from build123d import *

# Parameters (mm, degrees)
SKETCH1_W           = 90
SKETCH1_H           = 60
BOSS_EXTRUDE1_DEPTH = 5
SKETCH2_R           = 1.1
SKETCH2_R_2         = 0.62
SKETCH2_R_3         = 0.6858
SKETCH2_R_4         = 0.5
CUT_EXTRUDE1_DEPTH  = 61
SKETCH3_R           = 2
CUT_EXTRUDE2_DEPTH  = 6


with BuildPart() as part:
    # Sketch1 → Boss-Extrude1 (new body)
    with BuildSketch(Plane(origin=(0, 0, 0), x_dir=(1, 0, 0), z_dir=(0, 1, 0))):
        with Locations((-15.754716981, 62.075471698)):
            Rectangle(SKETCH1_W, SKETCH1_H)
    extrude(amount=BOSS_EXTRUDE1_DEPTH)

    # Sketch2 → Cut-Extrude1 (cut, through all)
    with BuildSketch(Plane.XY.offset(-32.075471698)):
        with Locations((-45.754716981, 5.25)):
            Circle(SKETCH2_R)
        with Locations((-25.754716981, 5.25)):
            Circle(SKETCH2_R_2)
        with Locations((-5.754716981, 5.25)):
            Circle(SKETCH2_R_3)
        with Locations((14.245283019, 5.25)):
            Circle(SKETCH2_R_4)
    extrude(amount=-CUT_EXTRUDE1_DEPTH, mode=Mode.SUBTRACT)

    # Sketch3 → Cut-Extrude2 (cut, through all)
    with BuildSketch(Plane(origin=(0, 5, 0), x_dir=(1, 0, 0), z_dir=(0, 1, 0))):
        with Locations((-53.907444579, 80.442311963)):
            Circle(SKETCH3_R)
        with Locations((-43.907444579, 80.442311963)):
            Circle(SKETCH3_R)
    extrude(amount=-CUT_EXTRUDE2_DEPTH, mode=Mode.SUBTRACT)


solid = part.part
Geometry check sheet. Reference: the model listing, model coordinates, mm. Round coordinates to 2 decimals unless told otherwise and drop trailing zeros. Write each loop counter-clockwise with the first axis right and the second up, starting at its lowest first coordinate (ties: lowest second). Pieces come first, ordered by that corner, then holes. Notation, with made-up numbers: (50, 41) -> (65, 41) arc R27 cw to (65, 61) -> close; hole circle Ø7 at (20, -7.5). An arc over 180 degrees is marked (long way). One line per item, written item: value. Start each with the question number.
(1) Draft check along X on faces 1 (the flat face through (29.245, 2, -62)), 2 (the cylindrical face through (-55.382, 2.535, -81.794)), 3 (the flat face through (-16, 2, -32.075)). Enter one of: +X half, -X half, draft (parallel to the pull), parting line (faces both ways), or undercut.
(2) Scan lines: line 1 (X direction, y = 2.7, z = -81); line 2 (X direction, y = 4.25, z = -66.5); line 3 (X direction, y = 4.3, z = -35). Record each from-to range of solid material in increasing order. Write a range as [from, to].
(3) Cross-section at A-A, the plane x = -53. Record the cut outline in (y, z).
Answer:
1. face 1: +X half
1. face 2: undercut
1. face 3: draft
2. line 1: [-60.75, -55.83], [-51.99, -45.83], [-41.99, 29.25]
2. line 2: [-60.75, -46.21], [-45.3, 29.25]
2. line 3: [-60.75, -46.31], [-45.2, 29.25]
3. outline: (0, -92.08) -> (5, -92.08) -> (5, -82.22) -> (0, -82.22) -> close; (0, -78.66) -> (5, -78.66) -> (5, -32.08) -> (0, -32.08) -> close
